For this review, take the finished solid that the model builds, in its own axes (mm). A direction names the side the tool comes from. Coordinates: 2 decimals unless noted, no trailing zeros. Write each loop counter-clockwise with the first axis right and the second up, starting at its lowest first coordinate (ties: lowest second). Pieces come first, ordered by that corner, then holes. Notation, with made-up numbers: (16.5, -28.75) -> (30.5, -28.75) arc R15 ccw to (30.5, -3.75) -> close; hole circle Ø1 at (4, 1.25). An arc over 180 degrees is marked (long way). Put each result on its own line as item: value. Start each with the question number.
Item 1: Consider section C-C on y = 75. Give the boundary of the cut face in (x, z).
Item 2: The part is to be moulded in two halves that separate along Y. For faces 1 (the flat face through (7, 140, 18)), 2 (the flat face through (28.965, 112.373, 17.745)), 3 (the cylindrical face through (11.832, 54.791, 21.893)), say which applies: +Y half, -Y half, draft (parallel to the pull), parting line (faces both ways), or undercut.
Item 3: Consider section A-A on z = 17.5. Give the number of separate pieces and of enclosed holes in the cut face, and give its area (3 significant figures).
Item 4: To check wall thickness, follow L1, parallel to Y at x = 17.75, z = 17.5; L2, parallel to Z at x = 9, y = 50; L3, parallel to Y at x = 9, z = 17.5. State the ranges of each line that lie inside material, in increasing order.
Item 5: Insertion check: P1, Ø12, axis at y = 115.5, z = 15.5, coming from the +X side; P2, Ø3, axis at x = 7.5, z = 16.5, coming from the +Y side; P3, Ø10.5, axis at y = 144.5, z = 12, coming from the -X side. Each pin has a flat end and moves straight along its axis. Give the tip position at first contact, or say it passes through.
Item 6: For faces 4 (the flat face through (0, 70, 17)), 5 (the flat face through (24, 69, 18)), list the 3-axis set-ups (+Z, -Z, +X, -X, +Y, -Y) from which the entire face can be reached by the end or side of a thin tool; tool diameter is ignored.
```python
from build123d import *

# Parameters (mm, degrees)
EXTRUDE_1_DEPTH        = 35
CUT_EXTRUDE_28_DEPTH   = 49
CUT_EXTRUDE_29_DEPTH   = 178.259696491
CUT_EXTRUDE_30_DEPTH   = 49
PATTERN_LINEAR_1_COUNT = 26
PATTERN_LINEAR_1_PITCH = 2
CHAMFER_2_SIZE         = 3.4
SKETCH_54_W            = 35
SKETCH_54_H            = 30
CUT_EXTRUDE_33_DEPTH   = 50
CUT_EXTRUDE_34_DEPTH   = 110
CHAMFER_3_SIZE         = 15
SKETCH_61_R            = 6.5
CUT_EXTRUDE_37_DEPTH   = 100
CUT_EXTRUDE_38_DEPTH   = 177.82480109
CUT_EXTRUDE_39_DEPTH   = 177.82480109


with BuildPart() as part:
    # 草图48 → 拉伸1 (new body)
    with BuildSketch(Plane.XY):
        Polygon((34.1, 110), (36, 110), (36, 0), (0, 0), (-0.0001, 170), (34.1, 170), (34.1, 144.543002638), align=None)
    extrude(amount=EXTRUDE_1_DEPTH)

    # 草图49 → 切除-拉伸28 (cut)
    with BuildSketch(Plane.XY.offset(35)):
        Polygon((34.1, 113.69999995), (29.174388239, 170), (34.1, 170), align=None)
    extrude(amount=-CUT_EXTRUDE_28_DEPTH, mode=Mode.SUBTRACT)

    # 草图50 → 切除-拉伸29 (cut, through all)
    with BuildSketch(Plane.XY.offset(35)):
        Polygon((27.668658483, 170), (29.261543982, 169.003805302), (29.174388239, 170), align=None)
    extrude(amount=-CUT_EXTRUDE_29_DEPTH, mode=Mode.SUBTRACT)

    # 草图51 → 切除-拉伸30 (cut)
    with BuildSketch(Plane.XY.offset(35)):
        Polygon((27.854407685, 167.876876901), (29.261543982, 169.003805302), (29.435855467, 167.011415906), align=None)
    cut_extrude_30 = extrude(amount=-CUT_EXTRUDE_30_DEPTH, mode=Mode.SUBTRACT)

    # 阵列(线性)1: 切除-拉伸30 ×26
    with Locations(*[Vector(0.08715574274765898, -0.9961946980917455, 0) * (i * PATTERN_LINEAR_1_PITCH) for i in range(1, PATTERN_LINEAR_1_COUNT)]):
        add(cut_extrude_30, mode=Mode.SUBTRACT)

    # 倒角2
    # the kernel refuses this chamfer: 3.4 mm, written as the material it takes off along each edge
    with BuildSketch(Plane(origin=(36, 110, -8.743722159), x_dir=(-0.9996219169112966, 0.027495876610587885, 0), z_dir=(0, 0, 1))) as chamfer_2_piece_1_section:
        Polygon((CHAMFER_2_SIZE * 0.999621916911, CHAMFER_2_SIZE * 0.0274958766106), (-CHAMFER_2_SIZE * 0.0274958766106, CHAMFER_2_SIZE * 0.999621916911), (0, 0), align=None)
    chamfer_2_piece_1 = extrude(amount=52.487444318, mode=Mode.PRIVATE)
    chamfer_2_piece_1 = split(chamfer_2_piece_1, bisect_by=Plane(origin=(34.1, 108.700122697, 17.5), z_dir=(1, 0, 0)), keep=Keep.TOP, mode=Mode.PRIVATE)
    add(chamfer_2_piece_1, mode=Mode.SUBTRACT)

    # 草图54 → 切除-拉伸33 (cut)
    with BuildSketch(Plane(origin=(36, 0, 0), x_dir=(0, 0, -1), z_dir=(1, 0, 0))):
        with Locations((-17.5, 15)):
            Rectangle(SKETCH_54_W, SKETCH_54_H)
    extrude(amount=-CUT_EXTRUDE_33_DEPTH, mode=Mode.SUBTRACT)

    # 草图56 → 切除-拉伸34 (cut)
    with BuildSketch(Plane.XY.offset(35)):
        Polygon((29, 106.6), (33.793642605, 117.201681001), (59.324325826, 70.82967178), (36, 30), (29, 30), align=None)
    extrude(amount=-CUT_EXTRUDE_34_DEPTH, mode=Mode.SUBTRACT)

    # 倒角3
    chamfer_3_edges = [part.edges().sort_by_distance(p)[0] for p in [
        (-0.0001, 170, 17.5),
    ]]
    chamfer(chamfer_3_edges, length=CHAMFER_3_SIZE)

    # 草图61 → 切除-拉伸37 (cut)
    with BuildSketch(Plane(origin=(0, 0, 0), x_dir=(0, 0, 1), z_dir=(-0.9999999999998271, -5.882352941191543e-07, 0))):
        with Locations(Location((17.5, 50, 0), (0, 0, 270))):
            Circle(SKETCH_61_R)
        with Locations(Location((17.5, 90, 0), (0, 0, 270))):
            Circle(SKETCH_61_R)
    extrude(amount=-CUT_EXTRUDE_37_DEPTH, mode=Mode.SUBTRACT)

    # 草图62 → 切除-拉伸38 (cut, through all)
    with BuildSketch(Plane.XY.offset(35)):
        Polygon((33.793642605, 117.201681001), (24, 107.408038396), (24, 30), (29, 30), (29, 106.6), align=None)
    extrude(amount=-CUT_EXTRUDE_38_DEPTH, mode=Mode.SUBTRACT)

    # 草图63 → 切除-拉伸39 (cut, through all)
    with BuildSketch(Plane.XY.offset(35)):
        Polygon((-6.5701e-05, 111.692243943), (6.999930181, 118.692239825), (6.999930181, 179.62094854), (-6.5701e-05, 176.661572218), (-12.74320746, 177.391313792), (-12.74320746, 111.692243943), align=None)
    extrude(amount=-CUT_EXTRUDE_39_DEPTH, mode=Mode.SUBTRACT)


solid = part.part
```
Return value:
1. outline: (0, 0) -> (24, 0) -> (24, 35) -> (0, 35) -> close
2. face 1: draft
2. face 2: -Y half
2. face 3: undercut
3. separate pieces: 3
3. enclosed holes: 0
3. area: 2,720 mm^2
4. L1: 30 to 43.5, 56.5 to 83.5, 96.5 to 170
4. L2: 0 to 11, 24 to 35
4. L3: 30 to 43.5, 56.5 to 83.5, 96.5 to 164
5. P1: x = 33.79
5. P2: y = 164
5. P3: x = 7
6. face 4: +Z, -Z, -X, +Y, -Y
6. face 5: +Z, -Z, +X, -Y
